Geometry check sheet. Reference: the model listing, model coordinates, mm. Give positions to 0.01 mm unless a question says otherwise; leave off trailing zeros. Write each loop counter-clockwise with the first axis right and the second up, starting at its lowest first coordinate (ties: lowest second). Pieces come first, ordered by that corner, then holes. Notation, with made-up numbers: M -8.75,-22.5 L 6.25,-22.5 A30 ccw 6.25,15.5 Z; hole C 11.5,65 d7. An arc over 180 degrees is marked long. Write each question's results on one line, items separated by ' | '.
```python
from build123d import *

# Parameters (mm, degrees)
SKETCH1_W           = 28.575
SKETCH1_H           = 33.655
BOSS_EXTRUDE1_DEPTH = 41.275
FILLET1_R           = 10
CUT_EXTRUDE2_DEPTH  = 56.139979201


with BuildPart() as part:
    # Sketch1 → Boss-Extrude1 (new, symmetric)
    with BuildSketch(Plane(origin=(0, 0, 0), x_dir=(0, 0, -1), z_dir=(1, 0, 0))):
        Rectangle(SKETCH1_W, SKETCH1_H)
    extrude(amount=BOSS_EXTRUDE1_DEPTH, both=True)

    # Fillet1
    fillet1_edges = [part.edges().sort_by_distance(p)[0] for p in [
        (41.275, 16.8275, 0),
        (-41.275, 16.8275, 0),
        (-41.275, -16.8275, 0),
        (41.275, -16.8275, 0),
    ]]
    fillet(fillet1_edges, radius=FILLET1_R)

    # Sketch2 → Cut-Extrude2 (cut, through all)
    with BuildSketch(Plane(origin=(0, 16.8275, 0), x_dir=(1, 0, 0), z_dir=(0, 1, 0))):
        with BuildLine():
            Line((-41.275, -9.573739396), (-47.491413454, -9.573739396))
            Line((-47.491413454, -9.573739396), (-47.491413454, -17.62428107))
            Line((-47.491413454, -17.62428107), (-24.575362808, -17.62428107))
            Line((-24.575362808, -17.62428107), (-24.575362808, -14.2875))
            add(Edge.make_bspline(
                [(-41.275, -9.573739396), (-36.608413477, -13.610536753), (-32.538276189, -14.2875), (-24.575362808, -14.2875)],
                knots=[0, 0, 0, 0, 1, 1, 1, 1], degree=3))
        make_face()
        with BuildLine():
            Line((24.575362808, -17.62428107), (24.575362808, -14.2875))
            add(Edge.make_bspline(
                [(41.275, -9.573739396), (36.608413477, -13.610536753), (32.538276189, -14.2875), (24.575362808, -14.2875)],
                knots=[0, 0, 0, 0, 1, 1, 1, 1], degree=3))
            Line((41.275, -9.573739396), (47.491413454, -9.573739396))
            Line((47.491413454, -9.573739396), (47.491413454, -17.62428107))
            Line((47.491413454, -17.62428107), (24.575362808, -17.62428107))
        make_face()
    extrude(amount=-CUT_EXTRUDE2_DEPTH, mode=Mode.SUBTRACT)


solid = part.part
```
Q1. Depth check by flat-ended pin: P1, Ø5, axis at y = -2.5, z = 10.5, coming from the -X side (3 decimals); P2, Ø1, axis at y = 1.5, z = 10.5, coming from the +X side. Enter the tip coordinate at first touch or a pass-through.
Answer key:
P1: stops at x = -41.275 | P2: stops at x = 40.77
Q2. Material ranges on probe 1 along Y at (x, z) = (36, -11.25); probe 2 along Z at (x, y) = (-28, 13); probe 3 along Z at (x, y) = (30.5, -7), recorded low to high. Write a range as [from, to].
Answer key:
probe 1: y = [-15.64, 15.64] | probe 2: z = [-14.29, 14.23] | probe 3: z = [-14.29, 14.06]
Q3. Section check A-A (z = 4). Enter the section's corners in (x, y) (1 decimal), then the cut area to 3 significant figures.
Answer key:
outline: M -41.3,-6.8 A10 ccw -31.3,-16.8 L 31.3,-16.8 A10 ccw 41.3,-6.8 L 41.3,6.8 A10 ccw 31.3,16.8 L -31.3,16.8 A10 ccw -41.3,6.8 Z | area: 2,690 mm2
